Build history of the part. All positions in model axes, mm. A direction names the side the tool comes from. Coordinates: 2 decimals unless noted, no trailing zeros. Loops run counter-clockwise (first coordinate to the right, second up) from the corner with the lowest first, then second, coordinate; pieces in that order, holes last.
(1) Wall check: L1, parallel to Y at x = 0, z = -11.6; L2, parallel to Y at x = 9, z = -5.5; L3, parallel to X at y = 16.5, z = -3. Give the ranges that are in metal, low to high.
(2) Slice it at C-C (z = -9). Give the cut face in (x, y).
(3) Tool access for faces 1 (the face through (5, -5, -13)), 2 (the face through (7, 0, -8)): list every direction of +Z, -Z, +X, -X, +Y, -Y with a clear straight run to the whole face (end or side of a thin tool).
(4) Two-plate mould, pull along X, no slides. Class faces 3 (the face through (23.846, 7.509, -6.409)), 4 (the face through (-2.222, -10.006, -6.226)), 5 (the face through (-17, 6, 0)): pulls with the +X half, pulls with the -X half, needs draft (parallel to the pull), parting line crosses it, or undercut.
(5) Flat gauge pins, fed straight in: P1, Ø4, axis at x = -13, y = -3, coming from the +Z side; P2, Ø10, axis at x = -3, y = -1, coming from the +Z side; P3, Ø3, axis at x = -11.5, z = -5, coming from the +Y side. Where does each tip first touch, or does it go through?
(6) Slice it at D-D (y = -12). Give the cut face in (x, z), and give its area (3 significant figures).
(7) Slice it at A-A (x = 0). Give the cut face in (y, z).
from build123d import *

# Parameters (mm, degrees)
CROQUIS1_R              = 25
SALIENTE_EXTRUIR1_DEPTH = 13
CROQUIS2_R              = 17.75
CORTAR_EXTRUIR1_DEPTH   = 4.5
CROQUIS3_R              = 10.25
CORTAR_EXTRUIR2_DEPTH   = 3.5
CORTAR_EXTRUIR3_REACH   = 38.249
CROQUIS4_R              = 6.5


with BuildPart() as part:
    # Croquis1 → Saliente-Extruir1 (new body)
    with BuildSketch(Plane.XY):
        Circle(CROQUIS1_R)
    extrude(amount=-SALIENTE_EXTRUIR1_DEPTH)

    # Croquis2 → Cortar-Extruir1 (cut)
    with BuildSketch(Plane.XY):
        Circle(CROQUIS2_R)
    extrude(amount=-CORTAR_EXTRUIR1_DEPTH, mode=Mode.SUBTRACT)

    # Croquis3 → Cortar-Extruir2 (cut)
    with BuildSketch(Plane.XY.offset(-4.5)):
        Circle(CROQUIS3_R)
    extrude(amount=-CORTAR_EXTRUIR2_DEPTH, mode=Mode.SUBTRACT)

    # Croquis4 → Cortar-Extruir3 (cut, up to next)
    with BuildSketch(Plane.XY.offset(-8), mode=Mode.PRIVATE) as cortar_extruir3_sk1:
        Circle(CROQUIS4_R)
    cortar_extruir3_tool1 = extrude(cortar_extruir3_sk1.sketch, amount=-CORTAR_EXTRUIR3_REACH, mode=Mode.PRIVATE) & part.part
    add(cortar_extruir3_tool1.solids().sort_by_distance((0, 0, -8))[0], mode=Mode.SUBTRACT)


solid = part.part
Response values:
1. L1: y = -25 to -6.5, 6.5 to 25
1. L2: y = -23.32 to -4.91, 4.91 to 23.32
1. L3: x = -18.78 to -6.54, 6.54 to 18.78
2. outline: circle Ø50 at (0, 0); hole circle Ø13 at (0, 0)
3. face 1: -Z, +X, -X, +Y, -Y
3. face 2: +Z
4. face 3: parting line crosses it
4. face 4: undercut
4. face 5: needs draft
5. P1: stops at z = -4.5
5. P2: stops at z = -8
5. P3: stops at y = 22.91
6. outline: (-21.93, -13) - (21.93, -13) - (21.93, 0) - (13.08, 0) - (13.08, -4.5) - (-13.08, -4.5) - (-13.08, 0) - (-21.93, 0) - close
6. area: 453 mm2
7. outline: (-25, -13) - (-6.5, -13) - (-6.5, -8) - (-10.25, -8) - (-10.25, -4.5) - (-17.75, -4.5) - (-17.75, 0) - (-25, 0) - close; (6.5, -13) - (25, -13) - (25, 0) - (17.75, 0) - (17.75, -4.5) - (10.25, -4.5) - (10.25, -8) - (6.5, -8) - close
